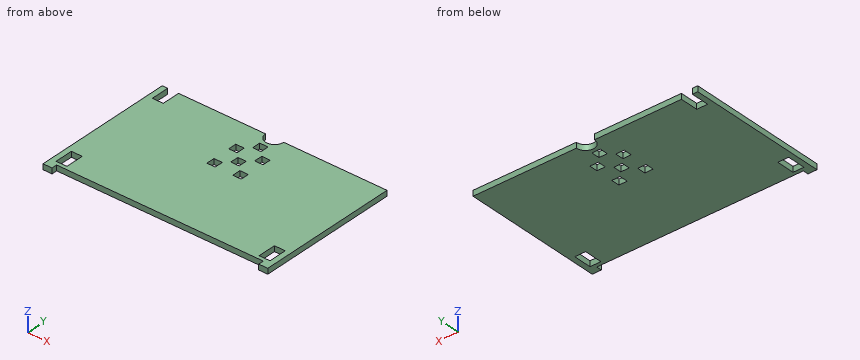
```python
from build123d import *

# Parameters (mm, degrees)
SKETCH1_W           = 6
SKETCH1_H           = 10
BOSS_EXTRUDE1_DEPTH = 3
SKETCH2_W           = 4.62
SKETCH2_H           = 4.62
CUT_EXTRUDE1_DEPTH  = 147.523035732


with BuildPart() as part:
    # Sketch1 → Boss-Extrude1 (new body)
    with BuildSketch(Plane.XY):
        with BuildLine():
            Line((0, 0), (5, 0))
            Line((5, 0), (5, 3))
            Line((5, 3), (119, 3))
            Line((119, 3), (119, 0))
            Line((119, 0), (124, 0))
            Line((124, 0), (124, 78))
            Line((124, 78), (67, 78))
            ThreePointArc((67, 78), (62, 73), (57, 78))
            Line((57, 78), (9, 78))
            Line((9, 78), (9, 68))
            Line((9, 68), (3, 68))
            Line((3, 68), (3, 78))
            Line((3, 78), (0, 78))
            Line((0, 78), (0, 0))
        make_face()
        with Locations((6, 10)):
            Rectangle(SKETCH1_W, SKETCH1_H, mode=Mode.SUBTRACT)
        with Locations((118, 10)):
            Rectangle(SKETCH1_W, SKETCH1_H, mode=Mode.SUBTRACT)
    extrude(amount=BOSS_EXTRUDE1_DEPTH)

    # Sketch2 → Cut-Extrude1 (cut, through all)
    with BuildSketch(Plane.XY.offset(3)):
        with Locations((54.84, 61.53)):
            Rectangle(SKETCH2_W, SKETCH2_H)
        with Locations((69.16, 61.53)):
            Rectangle(SKETCH2_W, SKETCH2_H)
        with Locations((54.84, 47.21)):
            Rectangle(SKETCH2_W, SKETCH2_H)
        with Locations((69.16, 47.21)):
            Rectangle(SKETCH2_W, SKETCH2_H)
        with Locations((62, 54.37)):
            Rectangle(SKETCH2_W, SKETCH2_H)
        with Locations((62, 68.69)):
            Rectangle(SKETCH2_W, SKETCH2_H)
    extrude(amount=-CUT_EXTRUDE1_DEPTH, mode=Mode.SUBTRACT)


solid = part.part
```
CAD build for the part. Positions are in the model's coordinates, mm. Coordinates: 2 decimals unless noted, no trailing zeros. Order: outer loops, then holes, each group sorted by start corner. A loop starts at its lowest first (then second) coordinate and runs counter-clockwise, first axis right, second up. Notation, with made-up numbers: M 60,65.25 L 66,65.25 A7 cw 66,77.25 Z; hole C 84,52.25 d7. An arc over 180 degrees is marked long. Write each question's results on one line, items separated by ' | '. Start each with the question number.
Q1. Cut at C-C (x = 105.5). List the corners of the cut face in (y, z), then the cut area to 3 significant figures.
Q2. Cut at B-B (z = 1.55). Count the separate pieces of the cut face and the enclosed holes in it, then the cut area to 3 significant figures.
Q3. Cut at A-A (x = 62). List the corners of the cut face in (y, z).
Q4. Drill centre lines: probe 1 along X at (y, z) = (9.5, 1.2); probe 2 along X at (y, z) = (69, 0.45); probe 3 along X at (y, z) = (67.5, 1.1). Where is each one in solid material? Low to high. Write a range as from..to.
Q5. Flat gauge pin, fed straight in: P1, Ø1.5, axis at x = 6, z = 1.5, coming from the +Y side. Where does the tip first touch, or does it go through?
Found:
1) outline: M 3,0 L 78,0 L 78,3 L 3,3 Z | area: 225 mm²
2) separate pieces: 1 | enclosed holes: 8 | area: 8,980 mm²
3) outline: M 3,0 L 52.06,0 L 52.06,3 L 3,3 Z; M 56.68,0 L 66.38,0 L 66.38,3 L 56.68,3 Z; M 71,0 L 73,0 L 73,3 L 71,3 Z
4) probe 1: 0..3, 9..115, 121..124 | probe 2: 0..3, 9..59.69, 64.31..124 | probe 3: 0..59.69, 64.31..124
5) P1: y = 68
